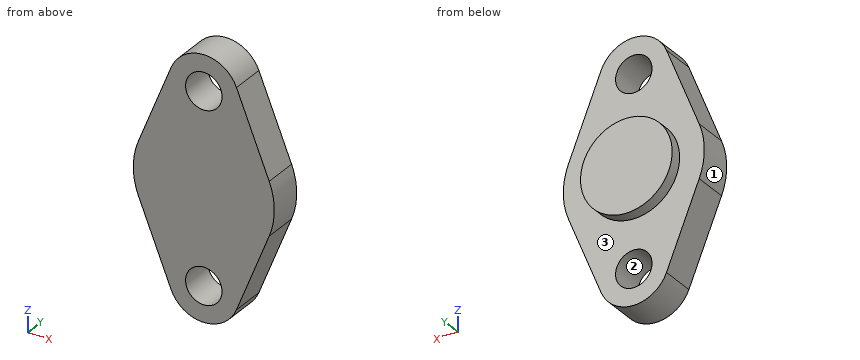
from build123d import *

# Parameters (mm, degrees)
CROQUIS2_R              = 1.55
SALIENTE_EXTRUIR1_DEPTH = 3
CROQUIS3_R              = 3.9
SALIENTE_EXTRUIR2_DEPTH = 1


with BuildPart() as part:
    # Croquis2 → Saliente-Extruir1 (new body)
    with BuildSketch(Plane(origin=(0, 0, 0), x_dir=(1, 0, 0), z_dir=(0, 1, 0))):
        with BuildLine():
            Line((2.781074433, 17.125), (5.562148865, 10.25))
            ThreePointArc((5.562148865, 10.25), (6, 8), (5.562148865, 5.75))
            Line((5.562148865, 5.75), (2.781074433, -1.125))
            ThreePointArc((2.781074433, -1.125), (0, -3), (-2.781074433, -1.125))
            Line((-2.781074433, -1.125), (-5.562148865, 5.75))
            ThreePointArc((-5.562148865, 5.75), (-6, 8), (-5.562148865, 10.25))
            Line((-5.562148865, 10.25), (-2.781074433, 17.125))
            ThreePointArc((-2.781074433, 17.125), (0, 19), (2.781074433, 17.125))
        make_face()
        with Locations((0, 16)):
            Circle(CROQUIS2_R, mode=Mode.SUBTRACT)
        Circle(CROQUIS2_R, mode=Mode.SUBTRACT)
    extrude(amount=SALIENTE_EXTRUIR1_DEPTH)

    # Croquis3 → Saliente-Extruir2 (add)
    with BuildSketch(Plane(origin=(0, 3, 0), x_dir=(1, 0, 0), z_dir=(0, 1, 0))):
        with Locations((0, 8)):
            Circle(CROQUIS3_R)
    extrude(amount=SALIENTE_EXTRUIR2_DEPTH)


solid = part.part
Geometry check sheet. Reference: the model listing, model coordinates, mm. Face numbers are marked on the shaded views. Coordinates: 2 decimals unless noted, no trailing zeros. Order: outer loops, then holes, each group sorted by start corner. A loop starts at its lowest first (then second) coordinate and runs counter-clockwise, first axis right, second up. Notation, with made-up numbers: (31.25, 18.5) -> (56.25, 18.5) arc R18 cw to (56.25, 45.5) -> close; hole circle Ø6 at (-31.5, 20). An arc over 180 degrees is marked (long way). Use a Markdown table: item, result. Add a question column.
1. Go/stop test with a flat-tipped pin: pin 1 Ø1.5 at (y, z) = (2.5, -0.5) entering from -X. Record where the tip stops, or that it passes through.
2. Mould release check, pull along Z, two halves, no side actions. Record for the marked faces 1, 2 and 3: pulls with the +Z half, pulls with the -Z half, needs draft (parallel to the pull), parting line crosses it, or undercut.
3. Cross-section at B-B (z = -16). Enter the section's corners in (x, y).
4. Material ranges on L1, parallel to Z at x = 0.5, y = 1.45; L2, parallel to Z at x = 0.75, y = 2; L3, parallel to Y at x = -1, z = -3, recorded low to high.
5. Cross-section at C-C (y = 2.65). Enter the section's corners in (x, z) (3 decimals), and give its area (3 significant figures).
6. Cross-section at A-A (x = 0). Enter the section's corners in (y, z), and give its area (3 significant figures).
7. Cross-section at D-D (z = -8). Enter the section's corners in (x, y).
Filled sheet:
| question | item | result |
|---|---|---|
| 1 | pin 1 | x = -3.74 |
| 2 | face 1 | parting line crosses it |
| 2 | face 2 | undercut |
| 2 | face 3 | needs draft |
| 3 | outline | (-3.24, 0) -> (-1.55, 0) -> (-1.55, 3) -> (-3.24, 3) -> close; (1.55, 0) -> (3.24, 0) -> (3.24, 3) -> (1.55, 3) -> close |
| 4 | L1 | -18.96 to -17.47, -14.53 to -1.47, 1.47 to 2.96 |
| 4 | L2 | -18.9 to -17.36, -14.64 to -1.36, 1.36 to 2.9 |
| 4 | L3 | 0 to 3 |
| 5 | outline | (-5.562, -10.25) -> (-2.781, -17.125) arc R3 ccw to (2.781, -17.125) -> (5.562, -10.25) arc R6 ccw to (5.562, -5.75) -> (2.781, 1.125) arc R3 ccw to (-2.781, 1.125) -> (-5.562, -5.75) arc R6 ccw to start; hole circle Ø3.1 at (0, -16); hole circle Ø3.1 at (0, 0) |
| 5 | area | 167 mm2 |
| 6 | outline | (0, -19) -> (3, -19) -> (3, -17.55) -> (0, -17.55) -> close; (0, -14.45) -> (3, -14.45) -> (3, -11.9) -> (4, -11.9) -> (4, -4.1) -> (3, -4.1) -> (3, -1.55) -> (0, -1.55) -> close; (0, 1.55) -> (3, 1.55) -> (3, 3) -> (0, 3) -> close |
| 6 | area | 55.2 mm2 |
| 7 | outline | (-6, 0) -> (6, 0) -> (6, 3) -> (3.9, 3) -> (3.9, 4) -> (-3.9, 4) -> (-3.9, 3) -> (-6, 3) -> close |
